The model under review builds one solid part; all positions refer to its coordinate system, in mm. A direction names the side the tool comes from. Coordinates: 2 decimals unless noted, no trailing zeros. Order: outer loops, then holes, each group sorted by start corner. A loop starts at its lowest first (then second) coordinate and runs counter-clockwise, first axis right, second up. Notation, with made-up numbers: M 36.25,50 L 75.25,50 A13 cw 75.25,68 Z; hole C 10.5,-10 d4. An arc over 180 degrees is marked long. One line per item, written item: value.
```python
from build123d import *

# Parameters (mm, degrees)
SKETCH007_R     = 52
PAD004_DEPTH    = 1.5
SKETCH008_R     = 25.5
POCKET001_DEPTH = 0.7
SKETCH010_W     = 8.4
SKETCH010_H     = 9
POCKET002_DEPTH = 10


with BuildPart() as part:
    # Sketch007 → Pad004 (new body, symmetric)
    with BuildSketch(Plane.XZ):
        Circle(SKETCH007_R)
    extrude(amount=PAD004_DEPTH, both=True)

    # Sketch008 (on Face2 of Pad004) → Pocket001 (cut)
    with BuildSketch(Plane(origin=(0, 1.5, 0), x_dir=(1, 0, 0), z_dir=(0, 1, 0))):
        Circle(SKETCH008_R)
    extrude(amount=-POCKET001_DEPTH, mode=Mode.SUBTRACT)

    # Sketch010 (on Face3 of Pocket001) → Pocket002 (cut)
    with BuildSketch(Plane.XZ.offset(1.5)):
        with Locations((0, -48.2)):
            Rectangle(SKETCH010_W, SKETCH010_H)
    extrude(amount=-POCKET002_DEPTH, mode=Mode.SUBTRACT)


solid = part.part
```
(1) Insertion check: pin 1 Ø10 at (x, z) = (-14, 16) entering from +Y; pin 2 Ø1 at (x, y) = (14.5, -1) entering from +Z; pin 3 Ø1.5 at (y, z) = (-1, 5) entering from -X. Each pin has a flat end and moves straight along its axis. Give the tip position at first contact, or say it passes through.
Geometry results:
pin 1: stops at y = 1.5
pin 2: stops at z = 50.08
pin 3: stops at x = -51.83
(2) For L1, parallel to Z at x = 0, y = 1.05; L2, parallel to X at y = 1.15, z = 0; L3, parallel to Y at x = -3.5, z = -16, list the stretches that pass through material, from the lowest coordinate up.
Geometry results:
L1: z = -43.7 to -25.5, 25.5 to 52
L2: x = -52 to -25.5, 25.5 to 52
L3: y = -1.5 to 0.8
(3) We need section B-B, the plane z = 0. State the section outline as (x, y) points.
Geometry results:
outline: M -52,-1.5 L 52,-1.5 L 52,1.5 L 25.5,1.5 L 25.5,0.8 L -25.5,0.8 L -25.5,1.5 L -52,1.5 Z
(4) We need section C-C, the plane y = -0.1. State the section outline as (x, z) points, plus the area to 3 significant figures.
Geometry results:
outline: M -4.2,-51.83 L -4.2,-43.7 L 4.2,-43.7 L 4.2,-51.83 A52 ccw long Z
area: 8,430 mm2
(5) We need section A-A, the plane x = 0. State the section outline as (y, z) points, plus the area to 3 significant figures.
Geometry results:
outline: M -1.5,-43.7 L 1.5,-43.7 L 1.5,-25.5 L 0.8,-25.5 L 0.8,25.5 L 1.5,25.5 L 1.5,52 L -1.5,52 Z
area: 251 mm2
(6) We need section D-D, the plane z = 27. State the section outline as (x, y) points.
Geometry results:
outline: M -44.44,-1.5 L 44.44,-1.5 L 44.44,1.5 L -44.44,1.5 Z
(7) Mouldability with a two-part tool opening along Z and no side actions: class faces 4 (the flat face through (-4.2, 0, -48)), 5 (the flat face through (0, 0, -43.7)), 6 (the flat face through (0, 0.8, 0)) as +Z half, -Z half, draft (parallel to the pull), parting line (faces both ways), or undercut.
Geometry results:
face 4: draft
face 5: -Z half
face 6: undercut
(8) Tool access review of faces 1 (the cylindrical face through (-5.5, 1.2, 24.9)), 2 (the flat face through (4.2, 0, -48)), 3 (the flat face through (11, 1.5, 24)): name each direction out of +Z, -Z, +X, -X, +Y, -Y from which nothing blocks a thin tool from reaching the whole face with its end or side.
Geometry results:
face 1: +Y
face 2: -Z, +Y, -Y
face 3: +Z, -Z, +X, -X, +Y
